Geometry: final body of the model. Coordinates: model frame, mm. Face numbers are marked on the shaded views. Coordinates: 2 decimals unless noted, no trailing zeros. One line per item, written item: value. Start each with the question number.
Item 1: Mould query, pull axis X, two halves, no side actions, for the marked faces 1 and 2. Classes: +X half, -X half, draft (parallel to the pull), parting line (faces both ways), or undercut.
Item 2: Ray query, probe 1 along Y at (x, z) = (0, 24); probe 2 along X at (y, z) = (23, 44); probe 3 along Z at (x, y) = (-22, 43). Return the intervals inside material, ascending. Write a range as from..to.
Item 3: Contact query for flat-ended pins moving along their axis: pin 1 Ø6 at (y, z) = (27.5, 38) entering from -X; pin 2 Ø1 at (x, z) = (4.5, 31.5) entering from -Y; pin 3 Ø3 at (x, y) = (-5, 35) entering from -Z; pin 4 Ø6 at (y, z) = (41.5, 75.5) entering from +X. Output: stop coordinate, or through.
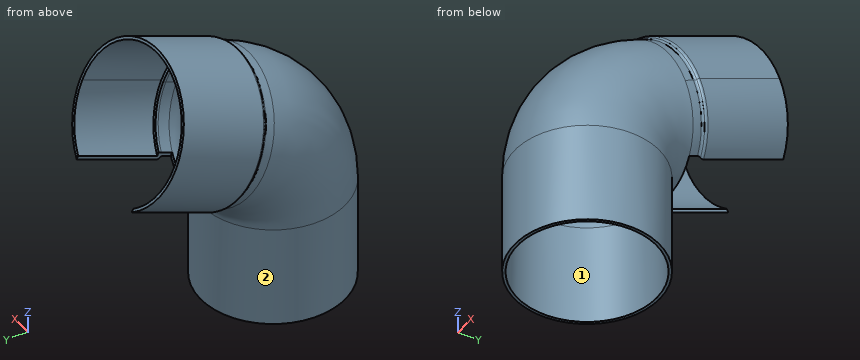
from build123d import *
from build123d.topology import SkipClean

# Parameters (mm, degrees)
ESQUISSE6_R             = 25
ESQUISSE6_R_2           = 24
ESQUISSE8_R             = 26
ESQUISSE8_R_2           = 24
EXTRU_MINCE1_DEPTH      = 1
EXTRU_MINCE2_START      = 30
ESQUISSE9_R             = 26
ESQUISSE9_R_2           = 25
EXTRU_MINCE2_DEPTH      = 30
CONG_1_R                = 1
CONG_2_R                = 1
ENL_V_MAT_EXTRU_1_DEPTH = 40


with BuildPart() as part:
    # Balayage-Mince2: sweep along a path in Esquisse7
    with BuildLine(Plane(origin=(0, 0, 0), x_dir=(0, 0, -1), z_dir=(1, 0, 0))) as balayage_mince2_path:
        Line((0, 0), (-35.14343316412919, -3.47e-15))
        ThreePointArc((-35.14343316412919, -3.47e-15), (-51.70154272349097, 4.983425337984965), (-62.75857876770245, 18.27806614532184))
        Line((-62.75857876770245, 18.27806614532184), (-64.37754708374251, 22.092116482858586))
    # Esquisse6 → Balayage-Mince2 (sweep)
    with BuildSketch(Plane.XY):
        Circle(ESQUISSE6_R)
        Circle(ESQUISSE6_R_2, mode=Mode.SUBTRACT)
    sweep(path=balayage_mince2_path.line)



with BuildPart() as body_2:
    # Esquisse8 → Extru.-Mince1 (new body)
    with BuildSketch(Plane(origin=(0, 41.87396099217143, 17.77444189612002), x_dir=(1, 0, 0), z_dir=(0, 0.9205048534524412, 0.39073112848927183))):
        with Locations((0, -50.62776693988426)):
            Circle(ESQUISSE8_R)
        with Locations((0, -50.62776693988426)):
            Circle(ESQUISSE8_R_2, mode=Mode.SUBTRACT)
    extrude(amount=EXTRU_MINCE1_DEPTH)


with BuildPart() as part_1:
    add(part.part)

    add(body_2.part)  # Extru.-Mince2 merges body 2
    # Esquisse9 → Extru.-Mince2 (add)
    with BuildSketch(Plane(origin=(0, 42.794465845623876, 18.16517302460929), x_dir=(1, 0, 0), z_dir=(0, 0.9205048534524412, 0.39073112848927183)).offset(EXTRU_MINCE2_START)):
        with Locations((0, -50.627766939884246)):
            Circle(ESQUISSE9_R)
        with Locations((0, -50.627766939884246)):
            Circle(ESQUISSE9_R_2, mode=Mode.SUBTRACT)
    extrude(amount=-EXTRU_MINCE2_DEPTH)

    # Congé1
    cong_1_edges = [part_1.edges().sort_by_distance(p)[0] for p in [
        (-25, 22.09211648285859, 64.3775470837425),
    ]]
    fillet(cong_1_edges, radius=CONG_1_R - 0.0001)  # a hair under: the kernel refuses the full size

    # Congé2
    cong_2_edges = [part_1.edges().sort_by_distance(p)[0] for p in [
        (-26, 22.092116482858604, 64.37754708374253),
    ]]
    fillet(cong_2_edges, radius=CONG_2_R)

    # Esquisse12 → Enlèv. mat.-Extru.1 (cut)
    with SkipClean():  # the faces are left unmerged after this step: merging them gives an invalid solid
        with BuildSketch(Plane(origin=(0, 0, 0), x_dir=(1, 0, 0), z_dir=(0, -0.39073112848927455, 0.9205048534524399))):
            Polygon((-15, 76.49021206691012), (15, 76.49021206691012), (15.000000000000004, 41.34677890278088), (-14.999999999999996, 41.34677890278088), align=None)
        extrude(amount=ENL_V_MAT_EXTRU_1_DEPTH, mode=Mode.SUBTRACT)


solid = part_1.part
Reply:
1. face 1: undercut
1. face 2: parting line
2. probe 1: y = -25..-24, 24..25
2. probe 2: x = -16.58..-15.03, 15.03..16.58
2. probe 3: z = 58.2..60.35, 86.15..88.31
3. pin 1: stops at x = -9.3
3. pin 2: stops at y = -24.68
3. pin 3: stops at z = 95.74
3. pin 4: stops at x = 26
